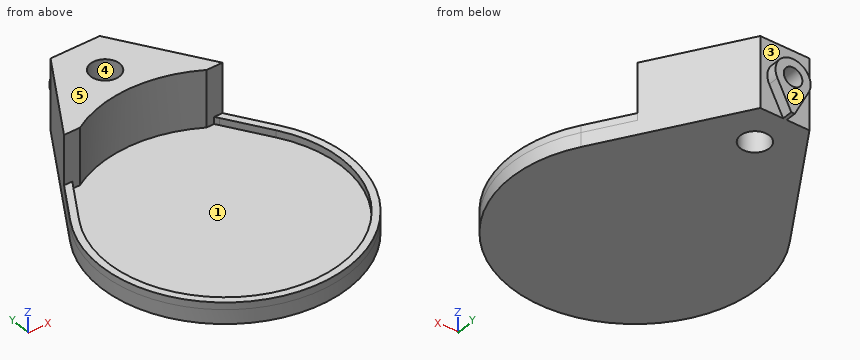
from build123d import *

# Parameters (mm, degrees)
CROQUIS1_R              = 35
SALIENTE_EXTRUIR1_DEPTH = 4
SALIENTE_EXTRUIR2_START = -4
CROQUIS2_R              = 4.1
SALIENTE_EXTRUIR2_DEPTH = 4
CROQUIS4_R              = 4.1
SALIENTE_EXTRUIR5_DEPTH = 16
CROQUIS7_W              = 70
CROQUIS7_H              = 60
CORTAR_EXTRUIR2_DEPTH   = 68.126745787
SALIENTE_EXTRUIR6_DEPTH = 2
CROQUIS12_R             = 2.65
SALIENTE_EXTRUIR8_DEPTH = 3
CORTAR_EXTRUIR5_START   = -16
CROQUIS13_R             = 2.65
CORTAR_EXTRUIR5_DEPTH   = 16


with BuildPart() as part:
    # Croquis1 → Saliente-Extruir1 (new body)
    with BuildSketch(Plane.XY):
        Circle(CROQUIS1_R)
    extrude(amount=SALIENTE_EXTRUIR1_DEPTH)

    # Croquis2 → Saliente-Extruir2 (add)
    with BuildSketch(Plane.XY.offset(4).offset(SALIENTE_EXTRUIR2_START)):
        with BuildLine():
            Line((29.716981132, 18.490566038), (7, 55))
            Line((7, 55), (-7, 55))
            Line((-7, 55), (-29.716981132, 18.490566038))
            ThreePointArc((-29.716981132, 18.490566038), (0, 35), (29.716981132, 18.490566038))
        make_face()
        with Locations((0, 44)):
            Circle(CROQUIS2_R, mode=Mode.SUBTRACT)
    extrude(amount=SALIENTE_EXTRUIR2_DEPTH)

    # Croquis4 → Saliente-Extruir5 (add)
    with BuildSketch(Plane.XY.offset(4)):
        with BuildLine():
            Line((29.716981132, 18.490566038), (7, 55))
            Line((7, 55), (-7, 55))
            Line((-7, 55), (-29.716981132, 18.490566038))
            ThreePointArc((-29.716981132, 18.490566038), (0, 35), (29.716981132, 18.490566038))
        make_face()
        with Locations((0, 44)):
            Circle(CROQUIS4_R, mode=Mode.SUBTRACT)
    extrude(amount=SALIENTE_EXTRUIR5_DEPTH)

    # Croquis7 → Cortar-Extruir2 (cut, through all)
    with BuildSketch(Plane.XY.offset(4)):
        Rectangle(CROQUIS7_W, CROQUIS7_H)
    extrude(amount=CORTAR_EXTRUIR2_DEPTH, mode=Mode.SUBTRACT)

    # Croquis8 → Saliente-Extruir6 (add)
    with BuildSketch(Plane.XY.offset(4)):
        with BuildLine():
            Line((-20.857442348, 28.943396226), (-28.018867925, 17.433962264))
            ThreePointArc((-28.018867925, 17.433962264), (0, -33), (28.018867925, 17.433962264))
            Line((28.018867925, 17.433962264), (20.857442348, 28.943396226))
            Line((20.857442348, 28.943396226), (20.2, 30))
            Line((20.2, 30), (22.555555556, 30))
            Line((22.555555556, 30), (29.716981132, 18.490566038))
            ThreePointArc((29.716981132, 18.490566038), (0, -35), (-29.716981132, 18.490566038))
            Line((-29.716981132, 18.490566038), (-22.555555556, 30))
            Line((-22.555555556, 30), (-20.2, 30))
            Line((-20.2, 30), (-20.857442348, 28.943396226))
        make_face()
    extrude(amount=SALIENTE_EXTRUIR6_DEPTH)

    # Croquis12 → Saliente-Extruir8 (add)
    with BuildSketch(Plane(origin=(0, 55, 0), x_dir=(1, 0, 0), z_dir=(0, 1, 0))):
        with BuildLine():
            Line((-4.451209869, -7.722560493), (-0.5, 0))
            Line((-0.5, 0), (0.5, 0))
            Line((0.5, 0), (4.451209869, -7.722560493))
            ThreePointArc((4.451209869, -7.722560493), (0, -15), (-4.451209869, -7.722560493))
        make_face()
        with Locations(Location((0, -10, 0), (0, 0, 270))):
            Circle(CROQUIS12_R, mode=Mode.SUBTRACT)
    extrude(amount=SALIENTE_EXTRUIR8_DEPTH)

    # Croquis13 → Cortar-Extruir5 (cut)
    with BuildSketch(Plane(origin=(0, 58, 0), x_dir=(1, 0, 0), z_dir=(0, 1, 0)).offset(CORTAR_EXTRUIR5_START)):
        with Locations(Location((0, -10, 0), (0, 0, 270))):
            Circle(CROQUIS13_R)
    extrude(amount=CORTAR_EXTRUIR5_DEPTH, mode=Mode.SUBTRACT)


solid = part.part
Model file for the job. Use its own axes, mm. Face numbers are marked on the shaded views. A direction names the side the tool comes from. Coordinates: 2 decimals unless noted, no trailing zeros. Write each loop counter-clockwise with the first axis right and the second up, starting at its lowest first coordinate (ties: lowest second). Pieces come first, ordered by that corner, then holes. Notation, with made-up numbers: (87, -39) - (113, -39) arc R17 cw to (113, -29) - close; hole circle Ø4 at (15.25, 83.5). An arc over 180 degrees is marked (long way). Write each question's results on one line, items separated by ' | '. Start each with the question number.
1) Cut at B-B (z = 16.5). Write the cut outline in (x, y).
2) Mould opens along Y. For the marked faces 3, 4 and 5 say: pulls with the +Y half, pulls with the -Y half, needs draft (parallel to the pull), parting line crosses it, or undercut.
3) 3-axis set-ups, long thin cutter, end or side, ignore diameter. For the marked faces 1 and 2: which of +Z, -Z, +X, -X, +Y, -Y reach the whole face in a straight line?
4) Cut at A-A (y = 43). Write the cut outline in (x, z), then the cut area to 3 significant figures.
5) Cut at C-C (y = 0). Write the cut outline in (x, z), then the cut area to 3 significant figures.
6) Cut at D-D (x = -25). Write the cut outline in (y, z).
7) Flat gauge pins, fed straight in: P1, Ø8, axis at x = -10.5, z = 3, coming from the +Y side; P2, Ø12, axis at x = 20, z = 8.5, coming from the +Y side; P3, Ø1.5, axis at x = 6, y = -14.5, coming from the +Z side. Where does each tip first touch, or does it go through?
8) Probe line 1 along Y through (x, z) = (0, 5); line 2 along X through (y, z) = (0, 4.85); line 3 along Z through (x, y) = (-12, -1.5). List the from-to ranges inside material, lowest first. Write a range as from..to.
Returned:
1) outline: (-22.56, 30) - (-18.03, 30) arc R35 cw to (18.03, 30) - (22.56, 30) - (7, 55) - (-7, 55) - close; hole circle Ø8.2 at (0, 44)
2) face 3: pulls with the +Y half | face 4: undercut | face 5: needs draft
3) face 1: +Z | face 2: +Z, -Z, +X, -X, +Y
4) outline: (-14.47, 0) - (-3.98, 0) - (-3.98, 20) - (-14.47, 20) - close; (3.98, 0) - (14.47, 0) - (14.47, 20) - (3.98, 20) - close | area: 420 mm^2
5) outline: (-35, 0) - (35, 0) - (35, 6) - (33, 6) - (33, 4) - (-33, 4) - (-33, 6) - (-35, 6) - close | area: 288 mm^2
6) outline: (-24.49, 0) - (26.07, 0) - (26.07, 6) - (22.29, 6) - (22.29, 4) - (-21.54, 4) - (-21.54, 6) - (-24.49, 6) - close
7) P1: y = 55 | P2: y = 43.75 | P3: z = 4
8) line 1: -35..-33, 35..39.9, 48.1..58 | line 2: -35..-33, 33..35 | line 3: 0..4
